from build123d import *

# Parameters (mm, degrees)
SKETCH1_R           = 1.5875
BOSS_EXTRUDE1_DEPTH = 9.525


with BuildPart() as part:
    # Sketch1 → Boss-Extrude1 (new body)
    with BuildSketch(Plane(origin=(0, 0, 0), x_dir=(1, 0, 0), z_dir=(0, 1, 0))):
        with BuildLine():
            Line((0, 0), (42.418, 0))
            Line((42.418, 0), (42.418, 42.418))
            Line((42.418, 42.418), (32.639, 42.418))
            Line((32.639, 42.418), (32.639, 21.209))
            ThreePointArc((32.639, 21.209), (21.209, 9.779), (9.779, 21.209))
            Line((9.779, 21.209), (9.779, 42.418))
            Line((9.779, 42.418), (0, 42.418))
            Line((0, 42.418), (0, 0))
        make_face()
        with Locations((5.715, 36.703)):
            Circle(SKETCH1_R, mode=Mode.SUBTRACT)
        with Locations((36.703, 36.703)):
            Circle(SKETCH1_R, mode=Mode.SUBTRACT)
        with Locations((36.703, 5.715)):
            Circle(SKETCH1_R, mode=Mode.SUBTRACT)
        with Locations((5.715, 5.715)):
            Circle(SKETCH1_R, mode=Mode.SUBTRACT)
    extrude(amount=BOSS_EXTRUDE1_DEPTH)


solid = part.part
The listing builds one solid part. Answer for the finished solid, in the listing's coordinates (mm). A direction names the side the tool comes from. Round coordinates to 2 decimals unless told otherwise and drop trailing zeros. Order: outer loops, then holes, each group sorted by start corner. A loop starts at its lowest first (then second) coordinate and runs counter-clockwise, first axis right, second up. Notation, with made-up numbers: (-9, -17) -> (2, -17) arc R25 cw to (2, 7) -> close; hole circle Ø8 at (43.25, -13). An arc over 180 degrees is marked (long way). Put each result on its own line as item: value.
Q1. Determine the mould class of faces 1 (the cylindrical face through (38.217, 4.696, -6.192)), 2 (the flat face through (38, 5, -42.418)), 3 (the flat face through (9.779, 5, -32)), 4 (the cylindrical face through (4.545, 4.696, -6.788)) for opening direction Z: pulls with the +Z half, pulls with the -Z half, needs draft (parallel to the pull), parting line crosses it, or undercut.
Results list:
face 1: undercut
face 2: pulls with the -Z half
face 3: needs draft
face 4: undercut
Q2. Which of the six approach directions +Z, -Z, +X, -X, +Y, -Y give full straight-line access (tool end or side, diameter ignored) to faces 5 (the flat face through (32.639, 5, -32)), 6 (the flat face through (21, 9.525, -7))?
Results list:
face 5: -Z, +Y, -Y
face 6: +Z, -Z, +X, -X, +Y
Q3. Section C-C, the plane y = 3.5 is taken. Write down the section's boundary in (x, z) (1 decimal).
Results list:
outline: (0, -42.4) -> (9.8, -42.4) -> (9.8, -21.2) arc R11.4 cw to (32.6, -21.2) -> (32.6, -42.4) -> (42.4, -42.4) -> (42.4, 0) -> (0, 0) -> close; hole circle Ø3.2 at (5.7, -36.7); hole circle Ø3.2 at (5.7, -5.7); hole circle Ø3.2 at (36.7, -36.7); hole circle Ø3.2 at (36.7, -5.7)
Q4. Each of these flat-tipped pins is pushed along its axis until it touches: P1, Ø1.9, axis at x = 36.703, z = -36.703, coming from the -Y side; P2, Ø1, axis at x = 14.5, y = 6, coming from the -Z side. Where does it stop, or does it pass through?
Results list:
P1: through
P2: z = -12.34
Q5. Section A-A, the plane z = -26 is taken. Write down the section's boundary in (x, y) (3 decimals), and give its area (3 significant figures).
Results list:
outline: (0, 0) -> (9.779, 0) -> (9.779, 9.525) -> (0, 9.525) -> close; (32.639, 0) -> (42.418, 0) -> (42.418, 9.525) -> (32.639, 9.525) -> close
area: 186 mm^2
Q6. Section B-B, the plane x = 36 is taken. Write down the section's boundary in (y, z) (3 decimals), and give its area (3 significant figures).
Results list:
outline: (0, -42.418) -> (9.525, -42.418) -> (9.525, -38.126) -> (0, -38.126) -> close; (0, -35.28) -> (9.525, -35.28) -> (9.525, -7.138) -> (0, -7.138) -> close; (0, -4.292) -> (9.525, -4.292) -> (9.525, 0) -> (0, 0) -> close
area: 350 mm^2
Q7. Section D-D, the plane z = -37.5 is taken. Write down the section's boundary in (x, y) (3 decimals).
Results list:
outline: (0, 0) -> (4.342, 0) -> (4.342, 9.525) -> (0, 9.525) -> close; (7.088, 0) -> (9.779, 0) -> (9.779, 9.525) -> (7.088, 9.525) -> close; (32.639, 0) -> (35.33, 0) -> (35.33, 9.525) -> (32.639, 9.525) -> close; (38.076, 0) -> (42.418, 0) -> (42.418, 9.525) -> (38.076, 9.525) -> close
Q8. Consider line 1 along X through (y, z) = (1, -33.5); line 2 along Z through (x, y) = (35.5, 2); line 3 along X through (y, z) = (1.25, -6). Determine where each line is inside the solid, lowest interval first.
Results list:
line 1: 0 to 9.78, 32.64 to 42.42
line 2: -42.42 to -37.74, -35.67 to -6.75, -4.68 to 0
line 3: 0 to 4.15, 7.28 to 35.14, 38.26 to 42.42
